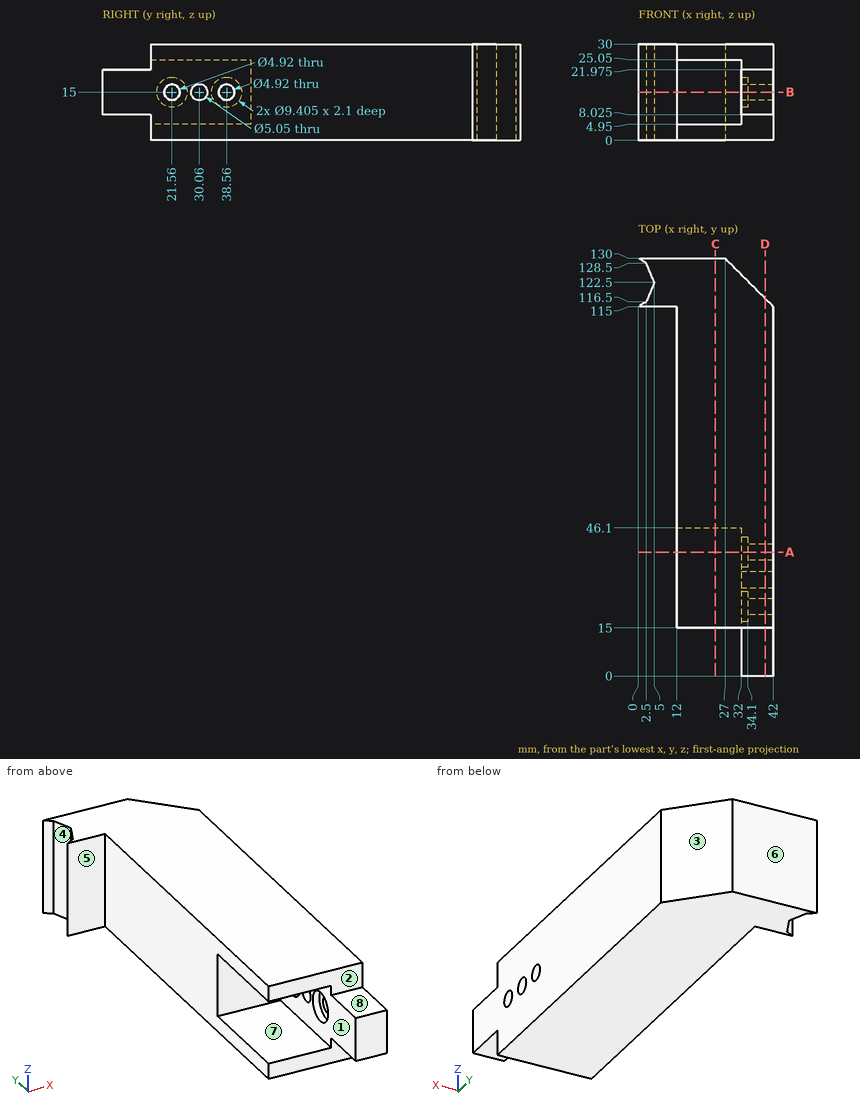
Answer from the drawing. Dimensions are ordinates in mm from the lowest x, y and z of the part. A direction names the side the tool comes from. Give positions to 0.01 mm unless a question says otherwise; leave off trailing zeros. Loops run counter-clockwise (first coordinate to the right, second up) from the corner with the lowest first, then second, coordinate; pieces in that order, holes last. Notation, with made-up numbers: M 4,-10.5 L 46,-10.5 A11 ccw 46,0.5 Z; hole C 14.5,22.5 d3. An arc over 180 degrees is marked long. One line per item, written item: value.
Q1. Find the intervals of material crossed by line 1 (Z direction, x = 27.5, y = 22); line 2 (Y direction, x = 39.5, z = 15) (3 decimals); line 3 (X direction, y = 82, z = 11.75), in increasing order. Write a range as from..to.
Working result:
line 1: z = 0..4.95, 25.05..30
line 2: y = 0..19.1, 24.02..27.535, 32.585..36.1, 41.02..117.5
line 3: x = 12..42
Q2. A cutting plane is placed at D-D on x = 39.5. Determine the outline of the cut face in (y, z) (3 decimals), then the cut area to 3 significant figures.
Working result:
outline: M 0,8.025 L 15,8.025 L 15,0 L 117.5,0 L 117.5,30 L 15,30 L 15,21.975 L 0,21.975 Z; hole C 21.56,15 d4.92; hole C 30.06,15 d5.05; hole C 38.56,15 d4.92
area: 3,230 mm^2
Q3. A cutting plane is placed at A-A on y = 38.56. Determine the outline of the cut face in (x, z).
Working result:
outline: M 12,0 L 42,0 L 42,12.54 L 34.1,12.54 L 34.1,10.3 L 32,10.3 L 32,4.95 L 12,4.95 Z; M 12,25.05 L 32,25.05 L 32,19.7 L 34.1,19.7 L 34.1,17.46 L 42,17.46 L 42,30 L 12,30 Z
Q4. Determine the mould class of the marked faces 6, 7 and 8 for opening direction Z: +Z half, -Z half, draft (parallel to the pull), parting line (faces both ways), or undercut.
Working result:
face 6: draft
face 7: undercut
face 8: +Z half
Q5. A cutting plane is placed at C-C on x = 24. Determine the outline of the cut face in (y, z).
Working result:
outline: M 15,0 L 130,0 L 130,30 L 15,30 L 15,25.05 L 46.1,25.05 L 46.1,4.95 L 15,4.95 Z
Q6. A cutting plane is placed at B-B on z = 15. Give the number of separate pieces and of enclosed holes in the cut face, then the cut area to 3 significant figures.
Working result:
separate pieces: 4
enclosed holes: 0
area: 2,830 mm^2
Q7. Flat-ended cylindrical pins translate along their axes: P1, Ø3, axis at y = 30.06, z = 15, coming from the -X side; P2, Ø10, axis at x = 26, z = 11.5, coming from the -Y side; P3, Ø2, axis at y = 33, z = 3.5, coming from the -X side; P4, Ø3, axis at x = 37.5, y = 8.5, coming from the -Z side (3 decimals). Find the tip coordinate at first contact, or state that the pin passes through.
Working result:
P1: passes through
P2: stops at y = 46.1
P3: stops at x = 12
P4: stops at z = 8.025
Q8. For the marked faces 1, 2, 3, 4 and 5, determine the directions among +Z, -Z, +X, -X, +Y, -Y from which every point of the face is accessible in a straight line to the end or side of a thin tool.
Working result:
face 1: -X, -Y
face 2: +Z, +X, -X, -Y
face 3: +Z, -Z, +X, +Y
face 4: +Z, -Z, -X
face 5: +Z, -Z, -X, -Y
